from build123d import *

# Parameters (mm, degrees)
SKETCH1_W           = 101.6
SKETCH1_H           = 304.8
BOSS_EXTRUDE1_DEPTH = 101.6
CUT_EXTRUDE1_DEPTH  = 101.6
SKETCH4_R           = 44.45
CUT_EXTRUDE2_DEPTH  = 508
SKETCH7_W           = 13.154000108
SKETCH7_H           = 13.97
CUT_EXTRUDE3_DEPTH  = 152.4
SKETCH8_W           = 101.6
SKETCH8_H           = 6.985
BOSS_EXTRUDE2_DEPTH = 6.35
CHAMFER1_SIZE       = 6.731
CHAMFER1_SIZE_2     = 11.658433986
SKETCH9_W           = 101.6
SKETCH9_H           = 292.826685396
BOSS_EXTRUDE3_DEPTH = 12.7
SKETCH10_W          = 101.6
SKETCH10_H          = 95.25
CUT_EXTRUDE4_DEPTH  = 58.42


with BuildPart() as part:
    # Sketch1 → Boss-Extrude1 (new body)
    with BuildSketch(Plane(origin=(0, 0, 0), x_dir=(1, 0, 0), z_dir=(0, 1, 0))):
        with Locations((50.8, -152.4)):
            Rectangle(SKETCH1_W, SKETCH1_H)
    extrude(amount=BOSS_EXTRUDE1_DEPTH)

    # Sketch3 → Cut-Extrude1 (cut)
    with BuildSketch(Plane(origin=(101.6, 0, 0), x_dir=(0, 0, -1), z_dir=(1, 0, 0))):
        Polygon((-304.8, 0), (0, 101.6), (-304.8, 101.6), align=None)
    extrude(amount=-CUT_EXTRUDE1_DEPTH, mode=Mode.SUBTRACT)

    # Sketch4 → Cut-Extrude2 (cut)
    with BuildSketch(Plane(origin=(0, 10.16, -30.48), x_dir=(-1, 0, 0), z_dir=(0, 0.31622776601683794, -0.9486832980505139))):
        with Locations((-50.8, 96.386223082)):
            Circle(SKETCH4_R)
    extrude(amount=-CUT_EXTRUDE2_DEPTH, mode=Mode.SUBTRACT)

    # Sketch7 → Cut-Extrude3 (cut)
    with BuildSketch(Plane(origin=(101.6, 0, 0), x_dir=(0, 0, -1), z_dir=(1, 0, 0))):
        with Locations((-15.213000054, 6.985)):
            Rectangle(SKETCH7_W, SKETCH7_H)
    extrude(amount=-CUT_EXTRUDE3_DEPTH, mode=Mode.SUBTRACT)

    # Sketch8 → Boss-Extrude2 (add)
    with BuildSketch(Plane.XY.offset(8.636)):
        with Locations((50.8, 3.4925)):
            Rectangle(SKETCH8_W, SKETCH8_H)
    extrude(amount=BOSS_EXTRUDE2_DEPTH)

    # Chamfer1
    # the kernel refuses this chamfer: 11.658433986, 6.731 mm, written as the material it takes off along each edge
    with BuildSketch(Plane(origin=(-30.161368486, 6.985, 14.986), x_dir=(0, 0.057893862402671366, -0.9983227437537926), z_dir=(1, 0, 0))) as chamfer1_piece_1_section:
        Polygon((CHAMFER1_SIZE * 0.998322743754, -CHAMFER1_SIZE * 0.0578938624027), (-CHAMFER1_SIZE_2 * 0.0578938624014, -CHAMFER1_SIZE_2 * 0.998322743732), (0, 0), align=None)
    chamfer1_piece_1 = extrude(amount=161.922736972, mode=Mode.PRIVATE)
    chamfer1_piece_1 = split(chamfer1_piece_1, bisect_by=Plane(origin=(50.8, 3.03450116, 8.636), z_dir=(0, 0, 1)), keep=Keep.TOP, mode=Mode.PRIVATE)
    add(chamfer1_piece_1, mode=Mode.SUBTRACT)

    # Sketch9 → Boss-Extrude3 (add)
    with BuildSketch(Plane.XZ):
        with Locations((50.8, 168.203342806)):
            Rectangle(SKETCH9_W, SKETCH9_H)
    extrude(amount=BOSS_EXTRUDE3_DEPTH)

    # Sketch10 → Cut-Extrude4 (cut)
    with BuildSketch(Plane(origin=(0, -12.7, 0), x_dir=(-1, 0, 0), z_dir=(0, -1, 0))):
        with Locations((-50.8, -266.991685504)):
            Rectangle(SKETCH10_W, SKETCH10_H)
    extrude(amount=-CUT_EXTRUDE4_DEPTH, mode=Mode.SUBTRACT)


solid = part.part
Model file for the job. Use its own axes, mm. A direction names the side the tool comes from. Give positions to 0.01 mm unless a question says otherwise; leave off trailing zeros. Order: outer loops, then holes, each group sorted by start corner. A loop starts at its lowest first (then second) coordinate and runs counter-clockwise, first axis right, second up. Notation, with made-up numbers: (34, 46.25) - (69, 46.25) arc R29 ccw to (69, 77.25) - close; hole circle Ø6 at (20, 35.25). An arc over 180 degrees is marked (long way). Return JSON: item names as keys, results as strings.
1) Cut at A-A, the plane x = 69.5. Give the cut face in (y, z).
Geometry says:
{"outline": "(-12.7, 21.79) - (13.97, 21.79) - (13.97, 8.64) - (6.33, 8.64) - (0, 12.29) - (0, 0) - (59.09, 0) - (0, 177.28) - (0, 219.37) - (-12.7, 219.37) - close"}
2) Pull direction Y, two halves, no side cores. Call faces 4 (the flat face through (3.219, 64.527, 111.219)), 5 (the flat face through (52, 13.97, 15)), 6 (the flat face through (50, 0, 6)): pulls with the +Y half, pulls with the -Y half, needs draft (parallel to the pull), parting line crosses it, or undercut.
Geometry says:
{"face 4": "pulls with the +Y half", "face 5": "undercut", "face 6": "pulls with the -Y half"}
3) Cut at B-B, the plane y = -2.5. Give the cut face in (x, z).
Geometry says:
{"outline": "(0, 21.79) - (101.6, 21.79) - (101.6, 219.37) - (0, 219.37) - close"}
4) Probe line 1 (Y direction, x = 65, z = 209); line 2 (X direction, y = 50, z = 60.5); line 3 (X direction, y = 77, z = 30.5). List the from-to ranges inside material, lowest first. Write a range as from..to.
Geometry says:
{"line 1": "-12.7..0", "line 2": "0..17.84, 83.76..101.6", "line 3": "0..8.51, 93.09..101.6"}
5) Cut at C-C, the plane x = 39.5. Give the cut face in (y, z), plus the area to 3 significant figures.
Geometry says:
{"outline": "(-12.7, 21.79) - (13.97, 21.79) - (13.97, 8.64) - (6.33, 8.64) - (0, 12.29) - (0, 0) - (56.28, 0) - (0, 168.85) - (0, 219.37) - (-12.7, 219.37) - close", "area": "7,090 mm²"}
6) Flat gauge pins, fed straight in: P1, Ø8, axis at x = 39, z = 133.5, coming from the +Y side; P2, Ø6, axis at x = 16.5, z = 55, coming from the +Y side; P3, Ø4, axis at x = 30.5, z = 17, coming from the -Y side. Where does each tip first touch, or does it go through?
Geometry says:
{"P1": "y = 13.8", "P2": "y = 57.88", "P3": "y = 13.97"}
7) 3-axis set-ups, long thin cutter, end or side, ignore diameter. For faces 1 (the flat face through (50, 1, 21.79)), 2 (the flat face through (52, 10, 8.636)), 3 (the flat face through (50, 0, 198)): which of +Z, -Z, +X, -X, +Y, -Y reach the whole face in a straight line?
Geometry says:
{"face 1": "+X, -X, -Y", "face 2": "+X, -X", "face 3": "+Z, +Y"}
